The model under review builds one solid part; all positions refer to its coordinate system, in mm. A direction names the side the tool comes from. Round coordinates to 2 decimals unless told otherwise and drop trailing zeros. Loops run counter-clockwise (first coordinate to the right, second up) from the corner with the lowest first, then second, coordinate; pieces in that order, holes last. Notation, with made-up numbers: (36.5, 20) -> (66.5, 20) arc R16 ccw to (66.5, 46) -> close; hole circle Ø4 at (7, 83.25). An arc over 180 degrees is marked (long way). Use CSV: the item, a comma, the result in double quotes. Start each with the question number.
```python
from build123d import *

# Parameters (mm, degrees)
SKETCH1_R           = 29.9974
SKETCH1_R_2         = 16
BOSS_EXTRUDE1_DEPTH = 7
SKETCH2_R           = 2
CUT_EXTRUDE1_DEPTH  = 10
SKETCH3_R           = 16
SKETCH3_R_2         = 15
BOSS_EXTRUDE2_DEPTH = 1
BOSS_EXTRUDE3_START = 3
SKETCH1_3_R         = 29.9974
SKETCH1_3_R_2       = 16
BOSS_EXTRUDE3_DEPTH = 3
BOSS_EXTRUDE4_START = 2
SKETCH3_2_R         = 16
SKETCH3_2_R_2       = 15
BOSS_EXTRUDE4_DEPTH = 2
SKETCH4_R           = 31.9974
SKETCH4_R_2         = 29.9974
BOSS_EXTRUDE5_DEPTH = 1
CUT_EXTRUDE3_START  = -1
SKETCH5_R           = 16
SKETCH5_R_2         = 15
CUT_EXTRUDE3_DEPTH  = 1
SKETCH6_R           = 3
SKETCH6_R_2         = 2
BOSS_EXTRUDE6_DEPTH = 3
CHAMFER1_SIZE       = 3
CUT_EXTRUDE4_START  = -10
SKETCH7_R           = 2
CUT_EXTRUDE4_DEPTH  = 10
BOSS_EXTRUDE7_START = 1
SKETCH8_R           = 16
SKETCH8_R_2         = 15
BOSS_EXTRUDE7_DEPTH = 1
CUT_EXTRUDE6_DEPTH  = 3


# Read off the part's stored shape, not the designer's step: Cut-Extrude5
with BuildPart() as part:
    # Sketch1 → Boss-Extrude1 (new body)
    with BuildSketch(Plane.XY):
        Circle(SKETCH1_R)
        Circle(SKETCH1_R_2, mode=Mode.SUBTRACT)
    extrude(amount=-BOSS_EXTRUDE1_DEPTH)

    # Sketch2 → Cut-Extrude1 (cut)
    with BuildSketch(Plane.XY):
        with Locations((25, 0)):
            Circle(SKETCH2_R)
        with Locations((0, -25)):
            Circle(SKETCH2_R)
        with Locations((-25, 0)):
            Circle(SKETCH2_R)
        with Locations((0, 25)):
            Circle(SKETCH2_R)
    extrude(amount=-CUT_EXTRUDE1_DEPTH, mode=Mode.SUBTRACT)

    # Sketch3 → Boss-Extrude2 (add)
    with BuildSketch(Plane.XY):
        Circle(SKETCH3_R)
        Circle(SKETCH3_R_2, mode=Mode.SUBTRACT)
    extrude(amount=-BOSS_EXTRUDE2_DEPTH)

    # Sketch1<3> → Boss-Extrude3 (add)
    with BuildSketch(Plane.XY.offset(BOSS_EXTRUDE3_START)):
        Circle(SKETCH1_3_R)
        Circle(SKETCH1_3_R_2, mode=Mode.SUBTRACT)
    extrude(amount=-BOSS_EXTRUDE3_DEPTH)

    # Sketch3<2> → Boss-Extrude4 (add)
    with BuildSketch(Plane.XY.offset(BOSS_EXTRUDE4_START)):
        Circle(SKETCH3_2_R)
        Circle(SKETCH3_2_R_2, mode=Mode.SUBTRACT)
    extrude(amount=-BOSS_EXTRUDE4_DEPTH)

    # Sketch4 → Boss-Extrude5 (add)
    with BuildSketch(Plane.XY.offset(3)):
        Circle(SKETCH4_R)
        Circle(SKETCH4_R_2, mode=Mode.SUBTRACT)
    extrude(amount=-BOSS_EXTRUDE5_DEPTH)

    # Sketch5 → Cut-Extrude3 (cut)
    with BuildSketch(Plane(origin=(0, 0, -1), x_dir=(-1, 0, 0), z_dir=(0, 0, -1)).offset(CUT_EXTRUDE3_START)):
        with Locations(Location((0, 0, 0), (0, 0, 180))):
            Circle(SKETCH5_R)
        with Locations(Location((0, 0, 0), (0, 0, 180))):
            Circle(SKETCH5_R_2, mode=Mode.SUBTRACT)
    extrude(amount=CUT_EXTRUDE3_DEPTH, mode=Mode.SUBTRACT)

    # Sketch6 → Boss-Extrude6 (add)
    # profile 1 of 4: a face of its own
    with BuildSketch(Plane(origin=(0, 0, -7), x_dir=(-1, 0, 0), z_dir=(0, 0, -1))):
        with Locations(Location((-25, 0, 0), (0, 0, 180))):
            Circle(SKETCH6_R)
        with Locations(Location((-25, 0, 0), (0, 0, 180))):
            Circle(SKETCH6_R_2, mode=Mode.SUBTRACT)
    # profile 2 of 4: a face of its own
    with BuildSketch(Plane(origin=(0, 0, -7), x_dir=(-1, 0, 0), z_dir=(0, 0, -1))):
        with Locations(Location((0, -25, 0), (0, 0, 180))):
            Circle(SKETCH6_R)
        with Locations(Location((0, -25, 0), (0, 0, 180))):
            Circle(SKETCH6_R_2, mode=Mode.SUBTRACT)
    # profile 3 of 4: a face of its own
    with BuildSketch(Plane(origin=(0, 0, -7), x_dir=(-1, 0, 0), z_dir=(0, 0, -1))):
        with Locations(Location((25, 0, 0), (0, 0, 180))):
            Circle(SKETCH6_R)
        with Locations(Location((25, 0, 0), (0, 0, 180))):
            Circle(SKETCH6_R_2, mode=Mode.SUBTRACT)
    # profile 4 of 4: a face of its own
    with BuildSketch(Plane(origin=(0, 0, -7), x_dir=(-1, 0, 0), z_dir=(0, 0, -1))):
        with Locations(Location((0, 25, 0), (0, 0, 180))):
            Circle(SKETCH6_R)
        with Locations(Location((0, 25, 0), (0, 0, 180))):
            Circle(SKETCH6_R_2, mode=Mode.SUBTRACT)
    extrude(amount=BOSS_EXTRUDE6_DEPTH)

    # Chamfer1
    # the kernel refuses this chamfer: 3 mm, written as the material it adds along each edge
    with BuildSketch(Plane(origin=(25, 0, -7), x_dir=(1, 0, 0), z_dir=(0, 1, 0))) as chamfer1_piece_1_section:
        Polygon((3 + CHAMFER1_SIZE, 0), (3, CHAMFER1_SIZE), (3, 0), align=None)
    chamfer1_piece_1 = revolve(axis=Axis((25, 0, -7), (0, 0, -1)), mode=Mode.PRIVATE)
    chamfer1_piece_1 = chamfer1_piece_1 & Plane(origin=(0, 0, -8.42256149), x_dir=(1, 0, 0), z_dir=(0, 0, 1)) * Cylinder(29.9974, 25, mode=Mode.PRIVATE)
    chamfer1_piece_1 = split(chamfer1_piece_1, bisect_by=Plane(origin=(20.492585696, 0, -10), z_dir=(0, 0, 1)), keep=Keep.TOP, mode=Mode.PRIVATE)
    add(chamfer1_piece_1)
    with BuildSketch(Plane(origin=(0, -25, -7), x_dir=(1, 0, 0), z_dir=(0, 1, 0))) as chamfer1_piece_2_section:
        Polygon((3 + CHAMFER1_SIZE, 0), (3, CHAMFER1_SIZE), (3, 0), align=None)
    chamfer1_piece_2 = revolve(axis=Axis((0, -25, -7), (0, 0, -1)), mode=Mode.PRIVATE)
    chamfer1_piece_2 = chamfer1_piece_2 & Plane(origin=(0, 0, -8.422561428), x_dir=(1, 0, 0), z_dir=(0, 0, 1)) * Cylinder(29.9974, 25, mode=Mode.PRIVATE)
    chamfer1_piece_2 = split(chamfer1_piece_2, bisect_by=Plane(origin=(-4.507414242, -25, -10), z_dir=(0, 0, 1)), keep=Keep.TOP, mode=Mode.PRIVATE)
    add(chamfer1_piece_2)
    with BuildSketch(Plane(origin=(-25, 0, -7), x_dir=(1, 0, 0), z_dir=(0, 1, 0))) as chamfer1_piece_3_section:
        Polygon((3 + CHAMFER1_SIZE, 0), (3, CHAMFER1_SIZE), (3, 0), align=None)
    chamfer1_piece_3 = revolve(axis=Axis((-25, 0, -7), (0, 0, -1)), mode=Mode.PRIVATE)
    chamfer1_piece_3 = chamfer1_piece_3 & Plane(origin=(0, 0, -8.422561427), x_dir=(1, 0, 0), z_dir=(0, 0, 1)) * Cylinder(29.9974, 25, mode=Mode.PRIVATE)
    chamfer1_piece_3 = split(chamfer1_piece_3, bisect_by=Plane(origin=(-29.507414241, 0, -10), z_dir=(0, 0, 1)), keep=Keep.TOP, mode=Mode.PRIVATE)
    add(chamfer1_piece_3)
    with BuildSketch(Plane(origin=(0, 25, -7), x_dir=(1, 0, 0), z_dir=(0, 1, 0))) as chamfer1_piece_4_section:
        Polygon((3 + CHAMFER1_SIZE, 0), (3, CHAMFER1_SIZE), (3, 0), align=None)
    chamfer1_piece_4 = revolve(axis=Axis((0, 25, -7), (0, 0, -1)), mode=Mode.PRIVATE)
    chamfer1_piece_4 = chamfer1_piece_4 & Plane(origin=(0, 0, -8.422561436), x_dir=(1, 0, 0), z_dir=(0, 0, 1)) * Cylinder(29.9974, 25, mode=Mode.PRIVATE)
    chamfer1_piece_4 = split(chamfer1_piece_4, bisect_by=Plane(origin=(-4.50741425, 25, -10), z_dir=(0, 0, 1)), keep=Keep.TOP, mode=Mode.PRIVATE)
    add(chamfer1_piece_4)

    # Sketch7 → Cut-Extrude4 (cut)
    with BuildSketch(Plane(origin=(0, 0, 0), x_dir=(-1, 0, 0), z_dir=(0, 0, -1)).offset(CUT_EXTRUDE4_START)):
        with Locations(Location((-25, 0, 0), (0, 0, 180))):
            Circle(SKETCH7_R)
        with Locations(Location((0, 25, 0), (0, 0, 180))):
            Circle(SKETCH7_R)
        with Locations(Location((25, 0, 0), (0, 0, 180))):
            Circle(SKETCH7_R)
        with Locations(Location((0, -25, 0), (0, 0, 180))):
            Circle(SKETCH7_R)
    extrude(amount=CUT_EXTRUDE4_DEPTH, mode=Mode.SUBTRACT)

    # Sketch8 → Boss-Extrude7 (add)
    with BuildSketch(Plane.XY.offset(2).offset(BOSS_EXTRUDE7_START)):
        Circle(SKETCH8_R)
        Circle(SKETCH8_R_2, mode=Mode.SUBTRACT)
    extrude(amount=-BOSS_EXTRUDE7_DEPTH)

    # Cut-Extrude5 outline → Cut-Extrude5 (revolve, cut)
    with BuildSketch(Plane(origin=(25, 0, 0), x_dir=(1, 0, 0), z_dir=(0, -1, 0))):
        Polygon((2, -7), (2, -10), (3, -10), (6, -7), align=None)
    revolve(axis=Axis((25, 0, 0), (0, 0, 1)), mode=Mode.SUBTRACT)

    # Cut-Extrude5 2 outline → Cut-Extrude5 2 (revolve, cut)
    with BuildSketch(Plane.XZ.offset(25)):
        Polygon((2, -7), (2, -10), (3, -10), (6, -7), align=None)
    revolve(axis=Axis((0, -25, 0), (0, 0, 1)), mode=Mode.SUBTRACT)

    # Cut-Extrude5 3 outline → Cut-Extrude5 3 (revolve, cut)
    with BuildSketch(Plane(origin=(-25, 0, 0), x_dir=(1, 0, 0), z_dir=(0, -1, 0))):
        Polygon((2, -7), (2, -10), (3, -10), (6, -7), align=None)
    revolve(axis=Axis((-25, 0, 0), (0, 0, 1)), mode=Mode.SUBTRACT)

    # Cut-Extrude5 4 outline → Cut-Extrude5 4 (revolve, cut)
    with BuildSketch(Plane.XZ.offset(-25)):
        Polygon((2, -7), (2, -10), (3, -10), (6, -7), align=None)
    revolve(axis=Axis((0, 25, 0), (0, 0, 1)), mode=Mode.SUBTRACT)

    # Sketch10 → Cut-Extrude6 (cut)
    with BuildSketch(Plane.XY.offset(3)):
        Polygon((-4.041451884, -25), (-2.020725942, -28.5), (2.020725942, -28.5), (4.041451884, -25), (2.020725942, -21.5), (-2.020725942, -21.5), align=None)
        Polygon((25, -4.041451884), (28.5, -2.020725942), (28.5, 2.020725942), (25, 4.041451884), (21.5, 2.020725942), (21.5, -2.020725942), align=None)
        Polygon((-25, 4.041451884), (-28.5, 2.020725942), (-28.5, -2.020725942), (-25, -4.041451884), (-21.5, -2.020725942), (-21.5, 2.020725942), align=None)
        Polygon((4.041451884, 25), (2.020725942, 28.5), (-2.020725942, 28.5), (-4.041451884, 25), (-2.020725942, 21.5), (2.020725942, 21.5), align=None)
    extrude(amount=-CUT_EXTRUDE6_DEPTH, mode=Mode.SUBTRACT)


solid = part.part
```
1. Clearance check with flat-ended pins moving along their axes: P1, Ø6.5, axis at x = 0, y = -25, coming from the +Z side; P2, Ø3.5, axis at x = -0.5, z = 1.5, coming from the -Y side; P3, Ø2, axis at y = 10.5, z = -1, coming from the +X side. State where each tip first meets the part, or that it passes through.
2. Take a section at C-C, the plane z = -4.75. Give the boundary of the cut face in (x, y).
3. Take a section at B-B, the plane x = 7. Give the boundary of the cut face in (y, z), then the cut area to 3 significant figures.
4. Take a section at A-A, the plane y = 0. Count the separate pieces of the cut face and the enclosed holes in it, then the cut area to 3 significant figures.
5. The part is to be moulded in two halves that separate along Y. For faces 3 (the face through (-29.97, 1.32, -2.44)), 4 (the face through (3.045, 26.726, 1.521)), 5 (the face through (13, -13, -7)), say which applies: pulls with the +Y half, pulls with the -Y half, needs draft (parallel to the pull), parting line crosses it, or undercut.
6. Take a section at D-D, the plane y = 10.5. Give the boundary of the cut face in (x, z).
7. For line 1 along Y through (x, z) = (0, -2.25); line 2 along X through (y, z) = (0, 1.6); line 3 along Y through (x, z) = (-3.5, 2.25), list the stretches that pass through material, from the lowest coordinate up. Write a range as from..to.
8. For faces 1 (the face through (0, -21.5, 2)), 2 (the face through (0.923, -23.226, -3.451)), list the 3-axis set-ups (+Z, -Z, +X, -X, +Y, -Y) from which the entire face can be reached by the end or side of a thin tool; tool diameter is ignored.
Results:
1,P1,"z = 0"
1,P2,"y = -32"
1,P3,"x = 28.45"
2,outline,"circle Ø59.99 at (0, 0); hole circle Ø4 at (-25, 0); hole circle Ø32 at (0, 0); hole circle Ø4 at (0, -25); hole circle Ø4 at (0, 25); hole circle Ø4 at (25, 0)"
3,outline,"(-31.22, 2) -> (-29.17, 2) -> (-29.17, -7) -> (-14.39, -7) -> (-14.39, 0) -> (-13.27, 0) -> (-13.27, 3) -> (-31.22, 3) -> close; (13.27, 0) -> (14.39, 0) -> (14.39, -7) -> (29.17, -7) -> (29.17, 2) -> (31.22, 2) -> (31.22, 3) -> (13.27, 3) -> close"
3,area,"306 mm²"
4,separate pieces,"4"
4,enclosed holes,"0"
4,area,"192 mm²"
5,face 3,"parting line crosses it"
5,face 4,"undercut"
5,face 5,"needs draft"
6,outline,"(-30.23, 2) -> (-28.1, 2) -> (-28.1, -7) -> (-12.07, -7) -> (-12.07, 0) -> (-10.71, 0) -> (-10.71, 3) -> (-30.23, 3) -> close; (10.71, 0) -> (12.07, 0) -> (12.07, -7) -> (28.1, -7) -> (28.1, 2) -> (30.23, 2) -> (30.23, 3) -> (10.71, 3) -> close"
7,line 1,"-30..-27, -23..-16, 16..23, 27..30"
7,line 2,"-30..-28.5, -21.5..-15, 15..21.5, 28.5..30"
7,line 3,"-31.81..-25.94, -24.06..-14.59, 14.59..24.06, 25.94..31.81"
8,face 1,"+Z"
8,face 2,"+Z, -Z"
